from build123d import *

# Parameters (mm, degrees)
SKETCH1_W           = 112.5
SKETCH1_H           = 24
BOSS_EXTRUDE1_DEPTH = 6
SKETCH2_W           = 8
SKETCH2_H           = 6
BOSS_EXTRUDE2_DEPTH = 6
SKETCH3_W           = 12
SKETCH3_H           = 6
BOSS_EXTRUDE3_DEPTH = 6


with BuildPart() as part:
    # Sketch1 → Boss-Extrude1 (new body)
    with BuildSketch(Plane(origin=(0, 0, 0), x_dir=(1, 0, 0), z_dir=(0, 1, 0))):
        Rectangle(SKETCH1_W, SKETCH1_H)
    extrude(amount=BOSS_EXTRUDE1_DEPTH)

    # Sketch2 → Boss-Extrude2 (add)
    with BuildSketch(Plane(origin=(0, 0, -12), x_dir=(-1, 0, 0), z_dir=(0, 0, -1))):
        with Locations((-18.75, 3)):
            Rectangle(SKETCH2_W, SKETCH2_H)
        with Locations((18.75, 3)):
            Rectangle(SKETCH2_W, SKETCH2_H)
    extrude(amount=BOSS_EXTRUDE2_DEPTH)

    # Sketch3 → Boss-Extrude3 (add)
    with BuildSketch(Plane.XY.offset(12)):
        with Locations((-38.25, 3)):
            Rectangle(SKETCH3_W, SKETCH3_H)
        with Locations((38.25, 3)):
            Rectangle(SKETCH3_W, SKETCH3_H)
    extrude(amount=BOSS_EXTRUDE3_DEPTH)


solid = part.part
Input: part model. Units: mm. Frame: model coordinates. A direction names the side the tool comes from. Coordinates: 2 decimals unless noted, no trailing zeros. Loops run counter-clockwise (first coordinate to the right, second up) from the corner with the lowest first, then second, coordinate; pieces in that order, holes last.
(1) Section C-C on z = 13. Return the cut outline in (x, y).
(2) Section B-B on y = 0.9. Return the cut outline in (x, z), then the cut area to 3 significant figures.
(3) First-contact query: pin 1 Ø1.8 at (y, z) = (2.5, -16.5) entering from +X; pin 2 Ø1.8 at (x, y) = (0, 3.5) entering from +Z; pin 3 Ø1.8 at (y, z) = (4.5, 15.5) entering from +X. Flat tips, straight axial feed; report the tip coordinate or a pass-through.
(4) Section A-A on z = -13.5. Return the cut outline in (x, y), then the cut area to 3 significant figures.
(5) Set-up query: faces 1 (the face through (22.75, 3, -15)), 2 (the face through (14.75, 3, -15)), 3 (the face through (-44.25, 3, 15)), 4 (the face through (-32.25, 3, 15)). Return all of +Z, -Z, +X, -X, +Y, -Y with unobstructed straight access to the full face (end or side cutting, diameter ignored); none if empty.
(6) Material intervals for probe 1 along X at (y, z) = (2.7, 16.5); probe 2 along X at (y, z) = (2.3, -14); probe 3 along Z at (x, y) = (26, 5.35), sorted ascending.
(7) Section D-D on x = -19. Return the cut outline in (y, z).
Data:
1. outline: (-44.25, 0) - (-32.25, 0) - (-32.25, 6) - (-44.25, 6) - close; (32.25, 0) - (44.25, 0) - (44.25, 6) - (32.25, 6) - close
2. outline: (-56.25, -12) - (-22.75, -12) - (-22.75, -18) - (-14.75, -18) - (-14.75, -12) - (14.75, -12) - (14.75, -18) - (22.75, -18) - (22.75, -12) - (56.25, -12) - (56.25, 12) - (44.25, 12) - (44.25, 18) - (32.25, 18) - (32.25, 12) - (-32.25, 12) - (-32.25, 18) - (-44.25, 18) - (-44.25, 12) - (-56.25, 12) - close
2. area: 2,940 mm2
3. pin 1: stops at x = 22.75
3. pin 2: stops at z = 12
3. pin 3: stops at x = 44.25
4. outline: (-22.75, 0) - (-14.75, 0) - (-14.75, 6) - (-22.75, 6) - close; (14.75, 0) - (22.75, 0) - (22.75, 6) - (14.75, 6) - close
4. area: 96.0 mm2
5. face 1: -Z, +X, +Y, -Y
5. face 2: -Z, +Y, -Y
5. face 3: +Z, -X, +Y, -Y
5. face 4: +Z, +Y, -Y
6. probe 1: x = -44.25 to -32.25, 32.25 to 44.25
6. probe 2: x = -22.75 to -14.75, 14.75 to 22.75
6. probe 3: z = -12 to 12
7. outline: (0, -18) - (6, -18) - (6, 12) - (0, 12) - close
